from build123d import *

# Parameters (mm, degrees)
ESQUISSE1_W              = 57
ESQUISSE1_H              = 57
BOSS_EXTRU_1_DEPTH       = 18.5
ESQUISSE2_W              = 51
ESQUISSE2_H              = 51
ENL_V_MAT_EXTRU_1_DEPTH  = 15.5
ESQUISSE4_W              = 10
ESQUISSE4_H              = 8
BOSS_EXTRU_2_DEPTH       = 10
ESQUISSE5_W              = 10
ESQUISSE5_H              = 8
BOSS_EXTRU_3_DEPTH       = 10
ESQUISSE6_W              = 10
ESQUISSE6_H              = 7
BOSS_EXTRU_4_DEPTH       = 10
ESQUISSE7_W              = 10
ESQUISSE7_H              = 7
BOSS_EXTRU_5_DEPTH       = 10
ESQUISSE8_R              = 1.7
ENL_V_MAT_EXTRU_2_DEPTH  = 12
ESQUISSE9_R              = 1.7
ENL_V_MAT_EXTRU_3_DEPTH  = 12
ESQUISSE16_R             = 1.7
ENL_V_MAT_EXTRU_9_DEPTH  = 12
ESQUISSE17_R             = 1.7
ENL_V_MAT_EXTRU_10_DEPTH = 12
ESQUISSE21_W             = 7.8
ESQUISSE21_H             = 2.8
ENL_V_MAT_EXTRU_14_DEPTH = 3
ENL_V_START              = -7.5
ENL_V_MAT_EXTRU_18_DEPTH = 2.7
ENL_V_MAT_EXTRU_20_DEPTH = 2.7
ESQUISSE26_W             = 5.54
ESQUISSE26_H             = 2.5
ENL_V_MAT_EXTRU_21_DEPTH = 2.847955181
ENL_V_MAT_EXTRU_22_DEPTH = 2.7
ENL_V_MAT_EXTRU_24_DEPTH = 2.7
ESQUISSE23_W             = 5.54
ESQUISSE23_H             = 2.5
ENL_V_MAT_EXTRU_26_DEPTH = 2
ESQUISSE31_W             = 5.54
ESQUISSE31_H             = 2.5
ENL_V_MAT_EXTRU_27_DEPTH = 2
ESQUISSE30_W             = 5.54
ESQUISSE30_H             = 2.5
ENL_V_MAT_EXTRU_28_DEPTH = 2
ESQUISSE32_W             = 57
ESQUISSE32_H             = 1
ENL_V_MAT_EXTRU_29_DEPTH = 0.5
ESQUISSE33_W             = 57
ESQUISSE33_H             = 1
ENL_V_MAT_EXTRU_30_DEPTH = 0.5
ESQUISSE34_W             = 57
ESQUISSE34_H             = 1
ENL_V_MAT_EXTRU_31_DEPTH = 0.5
ESQUISSE35_W             = 57
ESQUISSE35_H             = 1
ENL_V_MAT_EXTRU_32_DEPTH = 0.5
ESQUISSE36_W             = 11.4
ESQUISSE36_H             = 10.780005484
ENL_V_MAT_EXTRU_33_DEPTH = 2
CONG_1_R                 = 0.5
CONG_2_R                 = 0.5
CONG_3_R                 = 0.5
CONG_4_R                 = 0.5
CONG_5_R                 = 0.5
CONG_6_R                 = 0.5
CONG_7_R                 = 0.5
CONG_8_R                 = 0.5
CONG_9_R                 = 0.5
CONG_10_R                = 0.5
CONG_11_R                = 0.5
CONG_12_R                = 0.5


with BuildPart() as part:
    # Esquisse1 → Boss.-Extru.1 (new body)
    with BuildSketch(Plane(origin=(0, 0, 0), x_dir=(1, 0, 0), z_dir=(0, 1, 0))):
        with Locations((-1.510072399, 8.394175698)):
            Rectangle(ESQUISSE1_W, ESQUISSE1_H)
    extrude(amount=BOSS_EXTRU_1_DEPTH)

    # Esquisse2 → Enlèv. mat.-Extru.1 (cut)
    with BuildSketch(Plane(origin=(0, 18.5, 0), x_dir=(1, 0, 0), z_dir=(0, 1, 0))):
        with Locations((-1.510072399, 8.394175698)):
            Rectangle(ESQUISSE2_W, ESQUISSE2_H)
    extrude(amount=-ENL_V_MAT_EXTRU_1_DEPTH, mode=Mode.SUBTRACT)

    # Esquisse4 → Boss.-Extru.2 (add)
    with BuildSketch(Plane(origin=(0, 3, 0), x_dir=(1, 0, 0), z_dir=(0, 1, 0))):
        with Locations((-22.010072399, 29.894175698)):
            Rectangle(ESQUISSE4_W, ESQUISSE4_H)
    extrude(amount=BOSS_EXTRU_2_DEPTH)

    # Esquisse5 → Boss.-Extru.3 (add)
    with BuildSketch(Plane(origin=(0, 3, 0), x_dir=(1, 0, 0), z_dir=(0, 1, 0))):
        with Locations((18.989927601, 29.894175698)):
            Rectangle(ESQUISSE5_W, ESQUISSE5_H)
    extrude(amount=BOSS_EXTRU_3_DEPTH)

    # Esquisse6 → Boss.-Extru.4 (add)
    with BuildSketch(Plane(origin=(0, 3, 0), x_dir=(1, 0, 0), z_dir=(0, 1, 0))):
        with Locations((18.989927601, -13.605824302)):
            Rectangle(ESQUISSE6_W, ESQUISSE6_H)
    extrude(amount=BOSS_EXTRU_4_DEPTH)

    # Esquisse7 → Boss.-Extru.5 (add)
    with BuildSketch(Plane(origin=(0, 3, 0), x_dir=(1, 0, 0), z_dir=(0, 1, 0))):
        with Locations((-22.010072399, -13.605824302)):
            Rectangle(ESQUISSE7_W, ESQUISSE7_H)
    extrude(amount=BOSS_EXTRU_5_DEPTH)

    # Esquisse8 → Enlèv. mat.-Extru.2 (cut)
    with BuildSketch(Plane(origin=(0, 13, 0), x_dir=(1, 0, 0), z_dir=(0, 1, 0))):
        with Locations(Location((19.489927601, -13.105824302, 0), (0, 0, 270))):
            Circle(ESQUISSE8_R)
    extrude(amount=-ENL_V_MAT_EXTRU_2_DEPTH, mode=Mode.SUBTRACT)

    # Esquisse9 → Enlèv. mat.-Extru.3 (cut)
    with BuildSketch(Plane(origin=(0, 13, 0), x_dir=(1, 0, 0), z_dir=(0, 1, 0))):
        with Locations(Location((-22.510072399, -13.105824302, 0), (0, 0, 270))):
            Circle(ESQUISSE9_R)
    extrude(amount=-ENL_V_MAT_EXTRU_3_DEPTH, mode=Mode.SUBTRACT)

    # Esquisse16 → Enlèv. mat.-Extru.9 (cut)
    with BuildSketch(Plane(origin=(0, 13, 0), x_dir=(1, 0, 0), z_dir=(0, 1, 0))):
        with Locations(Location((-22.510072399, 28.894175698, 0), (0, 0, 270))):
            Circle(ESQUISSE16_R)
    extrude(amount=-ENL_V_MAT_EXTRU_9_DEPTH, mode=Mode.SUBTRACT)

    # Esquisse17 → Enlèv. mat.-Extru.10 (cut)
    with BuildSketch(Plane(origin=(0, 13, 0), x_dir=(1, 0, 0), z_dir=(0, 1, 0))):
        with Locations(Location((19.489927601, 28.894175698, 0), (0, 0, 270))):
            Circle(ESQUISSE17_R)
    extrude(amount=-ENL_V_MAT_EXTRU_10_DEPTH, mode=Mode.SUBTRACT)

    # Esquisse21 → Enlèv. mat.-Extru.14 (cut)
    with BuildSketch(Plane.XY.offset(20.105824302)):
        with Locations((-1.510072399, 16.07)):
            Rectangle(ESQUISSE21_W, ESQUISSE21_H)
    extrude(amount=-ENL_V_MAT_EXTRU_14_DEPTH, mode=Mode.SUBTRACT)

    # Esquisse24 → Enlèv. mat.-Extru.18 (cut)
    with BuildSketch(Plane(origin=(0, 13, 0), x_dir=(1, 0, 0), z_dir=(0, 1, 0)).offset(ENL_V_START)):
        Polygon((19.489927601, 25.694175698), (22.261208893, 27.294175698), (22.261208893, 30.494175698), (19.489927601, 32.094175698), (16.718646309, 30.494175698), (16.718646309, 27.294175698), align=None)
    extrude(amount=-ENL_V_MAT_EXTRU_18_DEPTH, mode=Mode.SUBTRACT)

    # Esquisse25 → Enlèv. mat.-Extru.20 (cut)
    with BuildSketch(Plane(origin=(0, 13, 0), x_dir=(1, 0, 0), z_dir=(0, 1, 0)).offset(ENL_V_START)):
        Polygon((16.718646309, -11.505824302), (16.718646309, -14.705824302), (19.489927601, -16.305824302), (22.261208893, -14.705824302), (22.261208893, -11.505824302), (19.489927601, -9.905824302), align=None)
    extrude(amount=-ENL_V_MAT_EXTRU_20_DEPTH, mode=Mode.SUBTRACT)

    # Esquisse26 → Enlèv. mat.-Extru.21 (cut)
    with BuildSketch(Plane(origin=(0, 0, 10.105824302), x_dir=(-1, 0, 0), z_dir=(0, 0, -1))):
        with Locations((-19.489927601, 4.25)):
            Rectangle(ESQUISSE26_W, ESQUISSE26_H)
    extrude(amount=-ENL_V_MAT_EXTRU_21_DEPTH, mode=Mode.SUBTRACT)

    # Esquisse27 → Enlèv. mat.-Extru.22 (cut)
    with BuildSketch(Plane(origin=(0, 13, 0), x_dir=(1, 0, 0), z_dir=(0, 1, 0)).offset(ENL_V_START)):
        Polygon((-19.738791107, 27.294175698), (-19.738791107, 30.494175698), (-22.510072399, 32.094175698), (-25.281353691, 30.494175698), (-25.281353691, 27.294175698), (-22.510072399, 25.694175698), align=None)
    extrude(amount=-ENL_V_MAT_EXTRU_22_DEPTH, mode=Mode.SUBTRACT)

    # Esquisse29 → Enlèv. mat.-Extru.24 (cut)
    with BuildSketch(Plane(origin=(0, 13, 0), x_dir=(1, 0, 0), z_dir=(0, 1, 0)).offset(ENL_V_START)):
        Polygon((-19.738791107, -11.505824302), (-22.510072399, -9.905824302), (-25.281353691, -11.505824302), (-25.281353691, -14.705824302), (-22.510072399, -16.305824302), (-19.738791107, -14.705824302), align=None)
    extrude(amount=-ENL_V_MAT_EXTRU_24_DEPTH, mode=Mode.SUBTRACT)

    # Esquisse23 → Enlèv. mat.-Extru.26 (cut)
    with BuildSketch(Plane.XY.offset(-25.894175698)):
        with Locations((19.489927601, 4.25)):
            Rectangle(ESQUISSE23_W, ESQUISSE23_H)
    extrude(amount=-ENL_V_MAT_EXTRU_26_DEPTH, mode=Mode.SUBTRACT)

    # Esquisse31 → Enlèv. mat.-Extru.27 (cut)
    with BuildSketch(Plane.XY.offset(-25.894175698)):
        with Locations((-22.510072399, 4.25)):
            Rectangle(ESQUISSE31_W, ESQUISSE31_H)
    extrude(amount=-ENL_V_MAT_EXTRU_27_DEPTH, mode=Mode.SUBTRACT)

    # Esquisse30 → Enlèv. mat.-Extru.28 (cut)
    with BuildSketch(Plane(origin=(0, 0, 10.105824302), x_dir=(-1, 0, 0), z_dir=(0, 0, -1))):
        with Locations((22.510072399, 4.25)):
            Rectangle(ESQUISSE30_W, ESQUISSE30_H)
    extrude(amount=-ENL_V_MAT_EXTRU_28_DEPTH, mode=Mode.SUBTRACT)

    # Esquisse32 → Enlèv. mat.-Extru.29 (cut)
    with BuildSketch(Plane.ZY.offset(30.010072399)):
        with Locations((-8.394175698, 8.219994516)):
            Rectangle(ESQUISSE32_W, ESQUISSE32_H)
    extrude(amount=-ENL_V_MAT_EXTRU_29_DEPTH, mode=Mode.SUBTRACT)

    # Esquisse33 → Enlèv. mat.-Extru.30 (cut)
    with BuildSketch(Plane.XY.offset(20.105824302)):
        with Locations((-1.510072399, 8.219994516)):
            Rectangle(ESQUISSE33_W, ESQUISSE33_H)
    extrude(amount=-ENL_V_MAT_EXTRU_30_DEPTH, mode=Mode.SUBTRACT)

    # Esquisse34 → Enlèv. mat.-Extru.31 (cut)
    with BuildSketch(Plane(origin=(26.989927601, 0, 0), x_dir=(0, 0, -1), z_dir=(1, 0, 0))):
        with Locations((8.394175698, 8.219994516)):
            Rectangle(ESQUISSE34_W, ESQUISSE34_H)
    extrude(amount=-ENL_V_MAT_EXTRU_31_DEPTH, mode=Mode.SUBTRACT)

    # Esquisse35 → Enlèv. mat.-Extru.32 (cut)
    with BuildSketch(Plane(origin=(0, 0, -36.894175698), x_dir=(-1, 0, 0), z_dir=(0, 0, -1))):
        with Locations((1.510072399, 8.219994516)):
            Rectangle(ESQUISSE35_W, ESQUISSE35_H)
    extrude(amount=-ENL_V_MAT_EXTRU_32_DEPTH, mode=Mode.SUBTRACT)

    # Esquisse36 → Enlèv. mat.-Extru.33 (cut)
    with BuildSketch(Plane.XY.offset(20.105824302)):
        with Locations((-1.510072399, 13.109997258)):
            Rectangle(ESQUISSE36_W, ESQUISSE36_H)
    extrude(amount=-ENL_V_MAT_EXTRU_33_DEPTH, mode=Mode.SUBTRACT)

    # Congé1
    cong_1_edges = [part.edges().sort_by_distance(p)[0] for p in [
        (-7.210072399, 13.609997258, 20.105824302),
    ]]
    fillet(cong_1_edges, radius=CONG_1_R)

    # Congé2
    cong_2_edges = [part.edges().sort_by_distance(p)[0] for p in [
        (4.189927601, 13.609997258, 20.105824302),
    ]]
    fillet(cong_2_edges, radius=CONG_2_R)

    # Congé3
    cong_3_edges = [part.edges().sort_by_distance(p)[0] for p in [
        (-7.210072399, 8.219994516, 19.605824302),
    ]]
    fillet(cong_3_edges, radius=CONG_3_R)

    # Congé4
    cong_4_edges = [part.edges().sort_by_distance(p)[0] for p in [
        (4.189927601, 8.219994516, 19.605824302),
    ]]
    fillet(cong_4_edges, radius=CONG_4_R)

    # Congé5
    cong_5_edges = [part.edges().sort_by_distance(p)[0] for p in [
        (26.989927601, 13.609997258, 20.105824302),
    ]]
    fillet(cong_5_edges, radius=CONG_5_R)

    # Congé6
    cong_6_edges = [part.edges().sort_by_distance(p)[0] for p in [
        (26.989927601, 3.859997258, 20.105824302),
    ]]
    fillet(cong_6_edges, radius=CONG_6_R)

    # Congé7
    cong_7_edges = [part.edges().sort_by_distance(p)[0] for p in [
        (26.989927601, 13.609997258, -36.894175698),
    ]]
    fillet(cong_7_edges, radius=CONG_7_R)

    # Congé8
    cong_8_edges = [part.edges().sort_by_distance(p)[0] for p in [
        (26.989927601, 3.859997258, -36.894175698),
    ]]
    fillet(cong_8_edges, radius=CONG_8_R)

    # Congé9
    cong_9_edges = [part.edges().sort_by_distance(p)[0] for p in [
        (-30.010072399, 13.609997258, -36.894175698),
    ]]
    fillet(cong_9_edges, radius=CONG_9_R)

    # Congé10
    cong_10_edges = [part.edges().sort_by_distance(p)[0] for p in [
        (-30.010072399, 3.859997258, -36.894175698),
    ]]
    fillet(cong_10_edges, radius=CONG_10_R)

    # Congé11
    cong_11_edges = [part.edges().sort_by_distance(p)[0] for p in [
        (-30.010072399, 13.609997258, 20.105824302),
    ]]
    fillet(cong_11_edges, radius=CONG_11_R)

    # Congé12
    cong_12_edges = [part.edges().sort_by_distance(p)[0] for p in [
        (-30.010072399, 3.859997258, 20.105824302),
    ]]
    fillet(cong_12_edges, radius=CONG_12_R)


solid = part.part
Read the model definition and answer for the solid it produces. Units are mm, in the model's axes. A direction names the side the tool comes from. Coordinates: 2 decimals unless noted, no trailing zeros. Write each loop counter-clockwise with the first axis right and the second up, starting at its lowest first coordinate (ties: lowest second). Pieces come first, ordered by that corner, then holes. Notation, with made-up numbers: M -29,-33 L 13,-33 A29 ccw 13,4 Z; hole C 21,-30 d9. An arc over 180 degrees is marked long. Use a Markdown table: item, result.
Q1. The part is cut by section C-C, the plane z = -3. Write down the section's boundary in (x, y), then the cut area to 3 significant figures.
Answer block:
| item | result |
|---|---|
| outline | M -30.01,0 L 26.99,0 L 26.99,7.72 L 26.49,7.72 L 26.49,8.72 L 26.99,8.72 L 26.99,18.5 L 23.99,18.5 L 23.99,3 L -27.01,3 L -27.01,18.5 L -30.01,18.5 L -30.01,8.72 L -29.51,8.72 L -29.51,7.72 L -30.01,7.72 Z |
| area | 263 mm2 |
Q2. Straight lines are drawn through the part: L1, parallel to X at y = 13, z = -9.5; L2, parallel to Z at x = 18.5, y = 17; L3, parallel to Z at x = -20.5, y = 9. For each, find the intervals that lie inside material, in ascending order. Write a range as [from, to].
Answer block:
| item | result |
|---|---|
| L1 | x = [-30.01, -27.01], [23.99, 26.99] |
| L2 | z = [-36.89, -33.89], [17.11, 20.11] |
| L3 | z = [-36.89, -25.89], [10.11, 20.11] |
Q3. The part is cut by section A-A, the plane x = -2.5. Write down the section's boundary in (y, z).
Answer block:
| item | result |
|---|---|
| outline | M 0,-36.89 L 7.72,-36.89 L 7.72,-36.39 L 8.72,-36.39 L 8.72,-36.89 L 18.5,-36.89 L 18.5,-33.89 L 3,-33.89 L 3,17.11 L 14.67,17.11 L 14.67,18.11 L 7.72,18.11 L 7.72,20.11 L 0,20.11 Z; M 17.47,17.11 L 18.5,17.11 L 18.5,18.11 L 17.47,18.11 Z |
Q4. The part is cut by section B-B, the plane y = 14. Write down the section's boundary in (x, z), then the cut area to 3 significant figures.
Answer block:
| item | result |
|---|---|
| outline | M -30.01,-36.39 A0.5 ccw -29.51,-36.89 L 26.49,-36.89 A0.5 ccw 26.99,-36.39 L 26.99,19.61 A0.5 ccw 26.49,20.11 L 4.69,20.11 A0.5 ccw 4.19,19.61 L 4.19,18.11 L -7.21,18.11 L -7.21,19.61 A0.5 ccw -7.71,20.11 L -29.51,20.11 A0.5 ccw -30.01,19.61 Z; hole M -27.01,-33.89 L 23.99,-33.89 L 23.99,17.11 L -27.01,17.11 Z |
| area | 625 mm2 |
Q5. The part is cut by section D-D, the plane y = 9.5. Give the number of separate pieces and of enclosed holes in the cut face, then the cut area to 3 significant figures.
Answer block:
| item | result |
|---|---|
| separate pieces | 1 |
| enclosed holes | 5 |
| area | 889 mm2 |
Q6. Each of these flat-tipped pins is pushed along its axis until it touches: pin 1 Ø5.5 at (y, z) = (8, 15) entering from -X; pin 2 Ø2 at (x, z) = (-10, -23.5) entering from +Y; pin 3 Ø3 at (x, y) = (-4, 11) entering from +Z. Where does it stop, or does it pass through?
Answer block:
| item | result |
|---|---|
| pin 1 | stops at x = -30.01 |
| pin 2 | stops at y = 3 |
| pin 3 | stops at z = 18.11 |
Q7. Which of the six approach directions +Z, -Z, +X, -X, +Y, -Y give full straight-line access (tool end or side, diameter ignored) to faces 1 (the face through (20, 1, -29)), 2 (the face through (-23.876, 4.169, -31.305))?
Answer block:
| item | result |
|---|---|
| face 1 | +Y |
| face 2 | none |
Q8. Determine the mould class of faces 3 (the face through (-23.92, 4.17, 15.49)), 4 (the face through (19, 5.5, -27)), 5 (the face through (-17.01, 8, 14)), 6 (the face through (-2, 18.5, -36)) for opening direction Y: released by +Y, released by -Y, zero draft, split by the parting line, or undercut.
Answer block:
| item | result |
|---|---|
| face 3 | undercut |
| face 4 | undercut |
| face 5 | zero draft |
| face 6 | released by +Y |
